Autodesk Inventor part; units mm, degrees
ref_plane "YZ Plane" through (0, 0, 0) normal (1, 0, 0) x (0, 1, 0)
ref_plane "XZ Plane" through (0, 0, 0) normal (0, 1, 0) x (-1, 0, 0)
ref_plane "XY Plane" through (0, 0, 0) normal (0, 0, 1) x (1, 0, 0)
sketch "Sketch1" plane through (0, 0, 0) normal (0, 1, 0) x (-1, 0, 0)
  circle A0 centre (0, 0) radius 47.5
  dimension "d0" = 95
extrude "Extrusion1" add sketch "Sketch1" along normal blind 6
sketch "Sketch2" plane through (0, 6, 0) normal (0, 1, 0) x (1, 0, 0)
  circle A0 centre (0, 0) radius 10
  circle A1 centre (0, 5) radius 1
  circle A2 centre (0, -5) radius 1
  dimension "d3" = 20
  dimension "d4" = 2
  dimension "d5" = 2
extrude "Extrusion2" cut sketch "Sketch2" against normal blind 23.4625 contours A1 | A2
sketch "Sketch3" plane through (0, 0, 0) normal (0, -1, 0) x (1, 0, 0)
  circle A0 centre (0, 0) radius 10
sketch "Sketch4" plane through (0, 6, 0) normal (0, 1, 0) x (1, 0, 0)
  line L0 (0, 0) -> (-10, 0)
  line L1 (-10, 0) -> (-10, 25)
  line L2 (-10, 25) -> (0, 25)
  line L3 (0, 25) -> (0, 0)
  line L4 (0, 0) -> (-5, 0)
  line L5 (-5, 0) -> (-5, 25)
  line L6 (-5, 25) -> (0, 25)
  line L7 (0, 25) -> (0, 0)
  line L8 (-5, 25) -> (-20, 25)
  line L9 (-20, 25) -> (-20, -25)
  line L10 (-20, -25) -> (-5, -25)
  line L11 (-5, -25) -> (-5, 25)
  line L12 (-5, 25) -> (-25, 25)
  line L13 (-25, 25) -> (-25, -25)
  line L14 (-25, -25) -> (-5, -25)
  line L15 (-5, -25) -> (-5, 25)
  dimension "d9" = 10
  dimension "d10" = 25
  dimension "d11" = 15
  dimension "d12" = 50
  dimension "d13" = 20
extrude "Extrusion3" add sketch "Sketch4" along normal blind 70 contours L11 L10 L9 L8 L1 L0 | L0 L1 L2 L5 | L14 L13 L12 L9
sketch "Sketch5" plane through (-25, 6, -25) normal (-1, 0, 0) x (0, 0, 1)
  line L0 (0, 0) -> (0, 70)
  line L1 (50, 0) -> (50, 70)
  line L2 (0, 70) -> (50, 70)
  line L3 (50, 70) -> (50, 0)
  line L4 (50, 0) -> (0, 0)
  line L5 (0, 0) -> (0, 70)
  line L6 (50, 70) -> (0, 70)
  line L7 (72.5, 0) -> (-22.5, 0)
  line L8 (0, 70) -> (25, 70)
  line L9 (25, 70) -> (25, 0)
  line L10 (25, 0) -> (0, 0)
  line L11 (0, 0) -> (0, 70)
  line L12 (25, 35) -> (15, 35)
  line L13 (15, 35) -> (15, 15)
  line L14 (15, 15) -> (25, 15)
  line L15 (25, 15) -> (25, 35)
  line L16 (15, 35) -> (25, 35)
  line L17 (25, 35) -> (25, 55)
  line L18 (25, 55) -> (15, 55)
  line L19 (15, 55) -> (15, 35)
  line L20 (15, 15) -> (35, 15)
  line L21 (35, 15) -> (35, 55)
  line L22 (35, 55) -> (15, 55)
  line L23 (15, 55) -> (15, 15)
  line L24 (15, 15) -> (35, 15)
  line L25 (35, 15) -> (35, 55.5)
  line L26 (35, 55.5) -> (15, 55.5)
  line L27 (15, 55.5) -> (15, 15)
  point P0 (25, -6)
  dimension "d16" = 10
  dimension "d17" = 20
  dimension "d18" = 20
  dimension "d19" = 20
  dimension "d20" = 40.5
extrude "Extrusion4" cut sketch "Sketch5" against normal blind 16 contours L14 L13 L12 L9 | L9 L22 L21 L20 | L26 L25 L22 L9 | L9 L18 L27 L26 | L12 L19 L18 L9
sketch "Sketch6" plane through (-25, 6, -25) normal (-1, 0, 0) x (0, 0, 1)
  line L0 (35, 15) -> (15, 15)
  line L1 (15, 15) -> (35, 15)
  line L2 (35, 15) -> (35, 9)
  line L3 (35, 9) -> (15, 9)
  line L4 (15, 9) -> (15, 15)
  line L5 (15, 55.5) -> (35, 55.5)
  line L6 (15, 55.5) -> (35, 55.5)
  line L7 (35, 55.5) -> (35, 61.5)
  line L8 (35, 61.5) -> (15, 61.5)
  line L9 (15, 61.5) -> (15, 55.5)
  point P0 (25, -6)
  dimension "d23" = 6
  dimension "d24" = 6
extrude "Extrusion5" cut sketch "Sketch6" against normal blind 6
sketch "Sketch7" plane through (-19, 6, -25) normal (-1, 0, 0) x (0, 0, 1)
  line L0 (35, 9) -> (15, 9)
  line L1 (35, 61.5) -> (35, 9)
  line L2 (15, 9) -> (35, 9)
  line L3 (35, 9) -> (35, 11.6)
  line L4 (35, 11.6) -> (15, 11.6)
  line L5 (15, 11.6) -> (15, 9)
  line L6 (15, 55.5) -> (15, 61.5)
  line L7 (35, 61.5) -> (35, 55.5)
  line L8 (15, 61.5) -> (35, 61.5)
  line L9 (35, 61.5) -> (35, 58.5)
  line L10 (35, 58.5) -> (15, 58.5)
  line L11 (15, 58.5) -> (15, 61.5)
  line L12 (15, 9) -> (15, 61.5)
  line L13 (15, 9) -> (35, 9)
  line L14 (35, 9) -> (35, 12)
  line L15 (35, 12) -> (15, 12)
  line L16 (15, 12) -> (15, 9)
  line L17 (35, 15) -> (15, 15)
  line L18 (25, 15) -> (20, 15)
  line L19 (20, 15) -> (20, 12)
  line L20 (20, 12) -> (25, 12)
  line L21 (25, 12) -> (25, 15)
  line L22 (25, 15) -> (30, 15)
  line L23 (30, 15) -> (30, 12)
  line L24 (30, 12) -> (25, 12)
  line L25 (25, 12) -> (25, 15)
  line L26 (15, 61.5) -> (35, 61.5)
  line L27 (25, 58.5) -> (20, 58.5)
  line L28 (20, 58.5) -> (20, 61.5)
  line L29 (20, 61.5) -> (25, 61.5)
  line L30 (25, 61.5) -> (25, 58.5)
  line L31 (25, 58.5) -> (30, 58.5)
  line L32 (30, 58.5) -> (30, 61.5)
  line L33 (30, 61.5) -> (25, 61.5)
  line L34 (25, 61.5) -> (25, 58.5)
  circle A0 centre (20, 12) radius 1.35
  circle A1 centre (30, 12) radius 1.35
  circle A2 centre (20, 58.5) radius 1.35
  circle A3 centre (30, 58.5) radius 1.35
  point P0 (25, -6)
  dimension "d27" = 2.6
  dimension "d28" = 3
  dimension "d29" = 3
  dimension "d30" = 5
  dimension "d31" = 5
  dimension "d32" = 2.7
  dimension "d33" = 2.7
  dimension "d34" = 2.7
  dimension "d35" = 2.7
extrude "Extrusion6" cut sketch "Sketch7" against normal blind 10 contours A1 L4 | L4 A1 L15 | A0 L15 L4 | L4 A0 | L15 L23 A1 | A0 L19 L15 | L15 A1 L23 | L15 L19 A0 | A3 L10 | L10 L32 A3 | A2 L28 L10 | L10 A2 | L10 A3 L32 | L28 A2 L10
thread "Thread1"
thread "Thread2"
thread "Thread3"
thread "Thread4"
sketch "Sketch8" plane through (-9, 6, -25) normal (-1, 0, 0) x (0, 0, 1)
  line L0 (15, 9) -> (15, 61.5)
  line L1 (35, 55.5) -> (35, 15)
  line L2 (15, 61.5) -> (35, 61.5)
  line L3 (35, 61.5) -> (35, 44.5)
  line L4 (35, 44.5) -> (15, 44.5)
  line L5 (15, 44.5) -> (15, 61.5)
  circle A0 centre (25, 44.5) radius 10
  point P0 (25, -6)
  dimension "d46" = 17
  dimension "d47" = 20
extrude "Extrusion7" cut sketch "Sketch8" against normal blind 15.4 contours A0 L4 | L4 A0
properties part number "NBase top"
Could you check a few things on this model? Use its own coordinates, in mm. A direction names the side the tool comes from. Round coordinates to 2 decimals unless told otherwise and drop trailing zeros. Loops run counter-clockwise (first coordinate to the right, second up) from the corner with the lowest first, then second, coordinate; pieces in that order, holes last.
Q1. I want a section at A-A (z = 0). Write out the boundary of the cut face in (x, y).
Q2. Thinking about a two-plate mould opening in Z: for faces 1 (the flat face through (-15, 41, 25)), 2 (the flat face through (1, 0, 1)), 3 (the flat face through (-9, 18, -5)), which applies, pulls with the +Z half, pulls with the -Z half, needs draft (parallel to the pull), parting line crosses it, or undercut?
Q3. On a 3-axis mill with a long thin cutter (end or side, diameter ignored), from which of +Z, -Z, +X, -X, +Y, -Y can I reach the whole of each face in a straight line? I mean faces 4 (the flat face through (-15, 41, -25)), 5 (the cylindrical face through (-14.07, 63.18, -5.29)), 6 (the flat face through (-25, 41, -11)). Say none if no direction works.
Q4. For P1, Ø23, axis at y = 50.5, z = 0, coming from the -X side; P2, Ø12, axis at y = 58, z = -1, coming from the -X side; P3, Ø6, axis at y = 33, z = -3, coming from the -X side, each with a flat end and sliding along its axis, tell me the tip position at first contact or that it passes through.
Q5. I want a section at C-C (y = 18). Write out the boundary of the cut face in (x, z), and give its area (3 significant figures).
Q6. Please list where these lines run through material, in increasing order: L1, parallel to Z at x = 0, y = 4.15; L2, parallel to Y at x = -12.75, z = -5; L3, parallel to Z at x = -11, y = 64.
Q7. I want a section at D-D (z = -16). Write out the boundary of the cut face in (x, y), and give its area (3 significant figures).
Q8. I want a section at B-B (y = 55). Write out the boundary of the cut face in (x, z).
Answer below:
1. outline: (-47.5, 0) - (47.5, 0) - (47.5, 6) - (-5, 6) - (-5, 40.5) - (-9, 40.5) - (-9, 21) - (-19, 21) - (-19, 15) - (-25, 15) - (-25, 6) - (-47.5, 6) - close; (-25, 67.5) - (-19, 67.5) - (-19, 61.5) - (-9, 61.5) - (-9, 60.5) - (-5, 60.5) - (-5, 76) - (-25, 76) - close
2. face 1: pulls with the +Z half
2. face 2: needs draft
2. face 3: undercut
3. face 4: -Z, +X, -X, +Y
3. face 5: -X
3. face 6: +Z, -Z, -X, +Y
4. P1: stops at x = -25
4. P2: stops at x = -19
4. P3: stops at x = -9
5. outline: (-25, -25) - (-5, -25) - (-5, 25) - (-25, 25) - (-25, 10) - (-19, 10) - (-19, 6.35) - (-9, 6.35) - (-9, 3.65) - (-19, 3.65) - (-19, -3.65) - (-9, -3.65) - (-9, -6.35) - (-19, -6.35) - (-19, -10) - (-25, -10) - close
5. area: 826 mm2
6. L1: z = -47.5 to -6, -4 to 4, 6 to 47.5
6. L2: y = 0 to 16.65, 19.35 to 21, 61.5 to 63.15, 65.85 to 76
6. L3: z = -25 to -6.25, -3.75 to 3.75, 6.25 to 25
7. outline: (-44.72, 0) - (44.72, 0) - (44.72, 6) - (-5, 6) - (-5, 76) - (-25, 76) - (-25, 6) - (-44.72, 6) - close
7. area: 1,940 mm2
8. outline: (-25, -25) - (-5, -25) - (-5, -8.93) - (-9, -8.93) - (-9, -10) - (-25, -10) - close; (-25, 10) - (-9, 10) - (-9, 8.93) - (-5, 8.93) - (-5, 25) - (-25, 25) - close
